from build123d import *

# Parameters (mm, degrees)
SKETCH1_W           = 20
SKETCH1_H           = 12
BOSS_EXTRUDE1_DEPTH = 20
SKETCH2_R           = 3
CUT_EXTRUDE1_DEPTH  = 13
SKETCH3_R           = 6.25
CUT_EXTRUDE2_DEPTH  = 4
SKETCH4_R           = 4.5
CUT_EXTRUDE3_DEPTH  = 9
SKETCH5_R           = 6.25
CUT_EXTRUDE4_DEPTH  = 4
BOSS_EXTRUDE2_DEPTH = 3
SKETCH7_R           = 6.25
CUT_EXTRUDE5_DEPTH  = 12
CHAMFER1_SIZE       = 6
CUT_EXTRUDE6_DEPTH  = 14
SKETCH9_W           = 3.789335489
SKETCH9_H           = 4.098961347
CUT_EXTRUDE7_DEPTH  = 2
SKETCH10_R          = 1.5
CUT_EXTRUDE8_DEPTH  = 4
CUT_EXTRUDE9_DEPTH  = 13
FILLET1_R           = 3


with BuildPart() as part:
    # Sketch1 → Boss-Extrude1 (new body)
    with BuildSketch(Plane.XY):
        with Locations((-59.5, -44)):
            Rectangle(SKETCH1_W, SKETCH1_H)
    extrude(amount=BOSS_EXTRUDE1_DEPTH)

    # Sketch2 → Cut-Extrude1 (cut, through all)
    with BuildSketch(Plane.XZ.offset(50)):
        with Locations((-59.5, 8)):
            Circle(SKETCH2_R)
    extrude(amount=-CUT_EXTRUDE1_DEPTH, mode=Mode.SUBTRACT)

    # Sketch3 → Cut-Extrude2 (cut)
    with BuildSketch(Plane.XZ.offset(50)):
        with Locations((-59.5, 8)):
            Circle(SKETCH3_R)
    extrude(amount=-CUT_EXTRUDE2_DEPTH, mode=Mode.SUBTRACT)

    # Sketch4 → Cut-Extrude3 (cut, through all)
    with BuildSketch(Plane.XZ.offset(46)):
        with Locations((-59.5, 8)):
            Circle(SKETCH4_R)
    extrude(amount=-CUT_EXTRUDE3_DEPTH, mode=Mode.SUBTRACT)

    # Sketch5 → Cut-Extrude4 (cut)
    with BuildSketch(Plane(origin=(0, -38, 0), x_dir=(1, 0, 0), z_dir=(0, 1, 0))):
        with Locations((-59.5, -8)):
            Circle(SKETCH5_R)
    extrude(amount=-CUT_EXTRUDE4_DEPTH, mode=Mode.SUBTRACT)

    # Sketch6 → Boss-Extrude2 (add)
    with BuildSketch(Plane(origin=(0, 0, 0), x_dir=(-1, 0, 0), z_dir=(0, 0, -1))):
        Polygon((49.5, -38), (41.5, -38), (41.5, -58), (77.5, -58), (77.5, -38), (69.5, -38), (69.5, -50), (49.5, -50), align=None)
    extrude(amount=-BOSS_EXTRUDE2_DEPTH)

    # Sketch7 → Cut-Extrude5 (cut)
    with BuildSketch(Plane.XZ.offset(58)):
        with Locations((-59.5, 8)):
            Circle(SKETCH7_R)
    extrude(amount=-CUT_EXTRUDE5_DEPTH, mode=Mode.SUBTRACT)

    # Chamfer1
    chamfer1_edges = [part.edges().sort_by_distance(p)[0] for p in [
        (-49.5, -44, 3),
        (-66.375, -50, 3),
        (-52.625, -50, 3),
        (-69.5, -44, 3),
    ]]
    chamfer(chamfer1_edges, length=CHAMFER1_SIZE)

    # Sketch8 → Cut-Extrude6 (cut)
    with BuildSketch(Plane.XY.offset(3)):
        Polygon((-47.645448267, -39.8), (-49.290896534, -42.65), (-47.645448267, -45.5), (-44.354551733, -45.5), (-42.709103466, -42.65), (-44.354551733, -39.8), align=None)
        Polygon((-47.645448267, -50.5), (-49.290896534, -53.35), (-47.645448267, -56.2), (-44.354551733, -56.2), (-42.709103466, -53.35), (-44.354551733, -50.5), align=None)
        Polygon((-74.645448267, -50.5), (-71.354551733, -50.5), (-69.709103466, -53.35), (-71.354551733, -56.2), (-74.645448267, -56.2), (-76.290896534, -53.35), align=None)
        Polygon((-74.645448267, -39.8), (-71.354551733, -39.8), (-69.709103466, -42.65), (-71.354551733, -45.5), (-74.645448267, -45.5), (-76.290896534, -42.65), align=None)
    extrude(amount=CUT_EXTRUDE6_DEPTH, mode=Mode.SUBTRACT)

    # Sketch9 → Cut-Extrude7 (cut)
    with BuildSketch(Plane.XY.offset(3)):
        with Locations((-43.394667744, -55.950519327)):
            Rectangle(SKETCH9_W, SKETCH9_H)
        with Locations((-75.605332256, -55.950519327)):
            Rectangle(SKETCH9_W, SKETCH9_H)
    extrude(amount=CUT_EXTRUDE7_DEPTH, mode=Mode.SUBTRACT)

    # Sketch10 → Cut-Extrude8 (cut, through all)
    with BuildSketch(Plane.XY.offset(3)):
        with Locations((-73, -42.65)):
            Circle(SKETCH10_R)
        with Locations((-73, -53.35)):
            Circle(SKETCH10_R)
        with Locations((-46, -53.35)):
            Circle(SKETCH10_R)
        with Locations((-46, -42.65)):
            Circle(SKETCH10_R)
    extrude(amount=-CUT_EXTRUDE8_DEPTH, mode=Mode.SUBTRACT)

    # Sketch11 → Cut-Extrude9 (cut, through all)
    with BuildSketch(Plane.XZ.offset(50)):
        with BuildLine():
            Line((-69.5, 20), (-69.5, 14.633249581))
            ThreePointArc((-69.5, 14.633249581), (-65.174548662, 18.573528147), (-59.5, 20))
            Line((-59.5, 20), (-69.5, 20))
        make_face()
        with BuildLine():
            ThreePointArc((-59.5, 20), (-53.825451338, 18.573528147), (-49.5, 14.633249581))
            Line((-49.5, 14.633249581), (-49.5, 20))
            Line((-49.5, 20), (-59.5, 20))
        make_face()
    extrude(amount=-CUT_EXTRUDE9_DEPTH, mode=Mode.SUBTRACT)

    # Fillet1
    fillet1_edges = [part.edges().sort_by_distance(p)[0] for p in [
        (-77.5, -58, 1.5),
        (-41.5, -58, 1.5),
    ]]
    fillet(fillet1_edges, radius=FILLET1_R)


solid = part.part
Geometry check sheet. Reference: the model listing, model coordinates, mm. A direction names the side the tool comes from. Give positions to 0.01 mm unless a question says otherwise; leave off trailing zeros. Loops run counter-clockwise (first coordinate to the right, second up) from the corner with the lowest first, then second, coordinate; pieces in that order, holes last.
(1) Section check D-D on x = -73. Record the cut outline in (y, z), then the cut area to 3 significant figures.
From the geometry:
outline: (-58, 0) - (-54.85, 0) - (-54.85, 3) - (-58, 3) - close; (-51.85, 0) - (-44.15, 0) - (-44.15, 3) - (-45.5, 3) - (-45.5, 5.5) - (-50.5, 5.5) - (-50.5, 3) - (-51.85, 3) - close; (-41.15, 0) - (-38, 0) - (-38, 5.5) - (-39.8, 5.5) - (-39.8, 3) - (-41.15, 3) - close
area: 59.0 mm2
(2) Set-up check for faces 4 (the flat face through (-64, -38, 3)), 5 (the flat face through (-69.5, -44, 12)), 6 (the flat face through (-48.71, -54.36, 4.01)), 7 (the flat face through (-73, -45.5, 5)), 8 (the flat face through (-46, -50.5, 5)): record each of +Z, -Z, +X, -X, +Y, -Y from which the full face is reachable in a straight line by a thin tool's end or side.
From the geometry:
face 4: +Z, -Z, +X, -X, +Y
face 5: +Z, -X, +Y, -Y
face 6: +Z, +X
face 7: +Z
face 8: +Z, -Y
(3) Section check C-C on y = -43.5. Record the cut outline in (x, z).
From the geometry:
outline: (-77.5, 0) - (-74.24, 0) - (-74.24, 3) - (-77.5, 3) - close; (-71.76, 0) - (-47.24, 0) - (-47.24, 3) - (-48.8, 3) - (-48.8, 8.3) - (-49.5, 9) - (-49.5, 14.63) arc R12 ccw to (-69.5, 14.63) - (-69.5, 9) - (-70.2, 8.3) - (-70.2, 3) - (-71.76, 3) - close; (-44.76, 0) - (-41.5, 0) - (-41.5, 3) - (-44.76, 3) - close; hole circle Ø9 at (-59.5, 8)
(4) Release check for a two-part mould opening along X. For faces 1 (the flat face through (-70.29, -54.36, 4.01)), 2 (the flat face through (-59, -58, 1)), 3 (the flat face through (-74.972, -44.935, 3.231)) record: released by +X, released by -X, zero draft, split by the parting line, or undercut.
From the geometry:
face 1: released by -X
face 2: zero draft
face 3: undercut
(5) Thickness scan on L1, parallel to Y at x = -73, z = 1; L2, parallel to X at y = -46.5, z = 13; L3, parallel to Z at x = -43.5, y = -50.25. Record the ranges inside material, lowest first.
From the geometry:
L1: y = -58 to -54.85, -51.85 to -44.15, -41.15 to -38
L2: x = -69.5 to -63.25, -55.75 to -49.5
L3: z = 0 to 3
(6) Section check A-A on y = -49.5. Record the cut outline in (x, z), then the cut area to 3 significant figures.
From the geometry:
outline: (-77.5, 0) - (-41.5, 0) - (-41.5, 3) - (-43.5, 3) - (-49.5, 9) - (-49.5, 14.63) arc R12 ccw to (-69.5, 14.63) - (-69.5, 9) - (-75.5, 3) - (-77.5, 3) - close; hole circle Ø12.5 at (-59.5, 8)
area: 329 mm2
(7) Section check B-B on x = -62.5. Record the cut outline in (y, z).
From the geometry:
outline: (-58, 0) - (-38, 0) - (-38, 2.52) - (-42, 2.52) - (-42, 4.65) - (-46, 4.65) - (-46, 2.52) - (-58, 2.52) - close; (-50, 13.48) - (-46, 13.48) - (-46, 11.35) - (-42, 11.35) - (-42, 13.48) - (-38, 13.48) - (-38, 19.62) - (-50, 19.62) - close
(8) Depth check by flat-ended pin: pin 1 Ø1.5 at (y, z) = (-46, 4) entering from +X; pin 2 Ø3.5 at (x, z) = (-46, 5.5) entering from -Y; pin 3 Ø1 at (y, z) = (-48, 11) entering from -X. Enter the tip coordinate at first touch or a pass-through.
From the geometry:
pin 1: stops at x = -43.75
pin 2: stops at y = -50.68
pin 3: stops at x = -69.5
